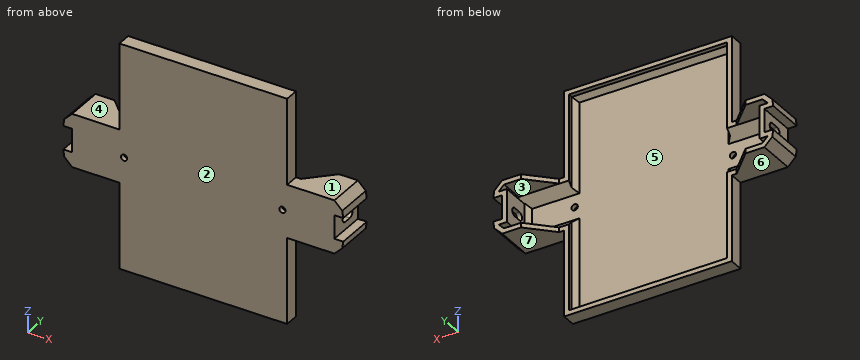
```python
from build123d import *

# Parameters (mm, degrees)
SKETCH4_W                = 90.422573022
SKETCH4_H                = 121.412
BOSS_EXTRUDE2_DEPTH      = 2.54
BOSS_EXTRUDE3_DEPTH      = 2.54
BOSS_EXTRUDE4_DEPTH      = 17.78
SKETCH7_W                = 121.034311438
SKETCH7_H                = 121.412
CUT_EXTRUDE1_DEPTH       = 12.7
CHAMFER1_SIZE            = 12.7
CHAMFER3_SIZE            = 5.08
CHAMFER4_SIZE            = 2.54
M4_START                 = -70.677155719
M4_CLEARANCE_SLOT1_DEPTH = 141.354311438
M3_CLEARANCE_HOLE1_D     = 3.4


# Read off the part's stored shape, not the designer's step: M4 Clearance Slot1
with BuildPart() as part:
    # Sketch4 → Boss-Extrude2 (new body)
    with BuildSketch(Plane(origin=(0, 0, 0), x_dir=(1, 0, 0), z_dir=(0, 1, 0))):
        Rectangle(SKETCH4_W, SKETCH4_H)
    extrude(amount=BOSS_EXTRUDE2_DEPTH)

    # Sketch5 → Boss-Extrude3 (add)
    with BuildSketch(Plane(origin=(0, 0, 0), x_dir=(1, 0, 0), z_dir=(0, 1, 0))):
        Polygon((45.211286511, 14.351), (70.694027546, 14.351), (74.922106204, 10.122921342), (75.452355719, 6.35), (70.677155719, 6.35), (70.677155719, -6.35), (75.452355719, -6.35), (74.922106204, -10.122921342), (70.694027546, -14.351), (45.211286511, -14.351), align=None)
        Polygon((-45.211286511, 14.351), (-45.211286511, -14.351), (-70.694027546, -14.351), (-74.922106204, -10.122921342), (-75.452355719, -6.35), (-70.677155719, -6.35), (-70.677155719, 6.35), (-75.452355719, 6.35), (-74.922106204, 10.122921342), (-70.694027546, 14.351), align=None)
    extrude(amount=BOSS_EXTRUDE3_DEPTH)

    # Sketch6 → Boss-Extrude4 (add)
    with BuildSketch(Plane(origin=(0, 2.54, 0), x_dir=(1, 0, 0), z_dir=(0, 1, 0))):
        Polygon((45.211286511, -60.706), (45.211286511, -14.351), (70.694027546, -14.351), (74.922106204, -10.122921342), (75.452355719, -6.35), (70.677155719, -6.35), (70.677155719, 6.35), (75.452355719, 6.35), (74.922106204, 10.122921342), (70.694027546, 14.351), (45.211286511, 14.351), (45.211286511, 60.706), (-45.211286511, 60.706), (-45.211286511, 14.351), (-70.694027546, 14.351), (-74.922106204, 10.122921342), (-75.452355719, 6.35), (-70.677155719, 6.35), (-70.677155719, -6.35), (-75.452355719, -6.35), (-74.922106204, -10.122921342), (-70.694027546, -14.351), (-45.211286511, -14.351), (-45.211286511, -60.706), align=None)
        Polygon((42.671286511, -58.166), (42.671286511, -11.811), (69.641925098, -11.811), (72.525104647, -8.927820451), (72.530419964, -8.89), (68.137155719, -8.89), (68.137155719, 8.89), (72.530419964, 8.89), (72.525104647, 8.927820451), (69.641925098, 11.811), (42.671286511, 11.811), (42.671286511, 58.166), (-42.671286511, 58.166), (-42.671286511, 11.811), (-69.641925098, 11.811), (-72.525104647, 8.927820451), (-72.530419964, 8.89), (-68.137155719, 8.89), (-68.137155719, -8.89), (-72.530419964, -8.89), (-72.525104647, -8.927820451), (-69.641925098, -11.811), (-42.671286511, -11.811), (-42.671286511, -58.166), align=None, mode=Mode.SUBTRACT)
    extrude(amount=BOSS_EXTRUDE4_DEPTH)

    # Sketch7 → Cut-Extrude1 (cut)
    with BuildSketch(Plane(origin=(0, 20.32, 0), x_dir=(1, 0, 0), z_dir=(0, 1, 0))):
        Rectangle(SKETCH7_W, SKETCH7_H)
    extrude(amount=-CUT_EXTRUDE1_DEPTH, mode=Mode.SUBTRACT)

    # Chamfer1
    chamfer1_edges = [part.edges().sort_by_distance(p)[0] for p in [
        (-60.517155719, 7.62, -13.081),
        (-60.517155719, 7.62, 13.081),
        (60.517155719, 7.62, 13.081),
        (60.517155719, 7.62, -13.081),
    ]]
    chamfer(chamfer1_edges, length=CHAMFER1_SIZE - 0.0001)  # a hair under: the kernel refuses the full size

    # Chamfer3
    chamfer3_edges = [part.edges().sort_by_distance(p)[0] for p in [
        (-56.156605804, 2.54, 11.811),
        (-56.156605804, 2.54, -11.811),
        (56.156605804, 2.54, 11.811),
        (56.156605804, 2.54, -11.811),
    ]]
    chamfer(chamfer3_edges, length=CHAMFER3_SIZE - 0.0001)  # a hair under: the kernel refuses the full size

    # Chamfer4
    chamfer4_edges = [part.edges().sort_by_distance(p)[0] for p in [
        (42.671286511, 2.54, 32.44855),
        (0, 2.54, 58.166),
        (-42.671286511, 2.54, 32.44855),
        (-42.671286511, 2.54, -32.44855),
        (42.671286511, 2.54, -32.44855),
        (0, 2.54, -58.166),
        (-68.137155719, 2.54, 0),
        (68.137155719, 2.54, 0),
    ]]
    chamfer(chamfer4_edges, length=CHAMFER4_SIZE)

    # M4 Clearance Slot1 outline → M4 Clearance Slot1 (cut)
    with BuildSketch(Plane.YZ.offset(M4_START)):
        with BuildLine():
            Line((9.43, -2.25), (13.43, -2.25))
            ThreePointArc((13.43, -2.25), (15.68, 0), (13.43, 2.25))
            Line((13.43, 2.25), (9.43, 2.25))
            ThreePointArc((9.43, 2.25), (7.18, 0), (9.43, -2.25))
        make_face()
    extrude(amount=M4_CLEARANCE_SLOT1_DEPTH, mode=Mode.SUBTRACT)

    # M3 Clearance Hole1 (through all)
    with Locations(Plane(origin=(0, 2.54, 0), x_dir=(1, 0, 0), z_dir=(0, 1, 0))):
        with Locations((42.671286511, 0), (-42.671286511, 0)):
            Hole(M3_CLEARANCE_HOLE1_D / 2)


solid = part.part
```
Model file for the job. Use its own axes, mm. Face numbers are marked on the shaded views. A direction names the side the tool comes from. Give positions to 0.01 mm unless a question says otherwise; leave off trailing zeros. Loops run counter-clockwise (first coordinate to the right, second up) from the corner with the lowest first, then second, coordinate; pieces in that order, holes last. Notation, with made-up numbers: (14.25, -20.5) - (51.25, -20.5) arc R26 cw to (51.25, 8.5) - close; hole circle Ø8 at (4.25, 57.5). An arc over 180 degrees is marked (long way). One line per item, written item: value. Start each with the question number.
1. Slice it at C-C (z = -20). List the corners of the cut face in (x, y).
2. Slice it at A-A (z = 0). List the corners of the cut face in (x, y), plus the area to 3 significant figures.
3. Slice it at B-B (x = -5.5). List the corners of the cut face in (y, z), plus the area to 3 significant figures.
4. Pin check, flat tips, straight feed: pin 1 (12 mm diameter, centred on y = 15.5, z = -1.5, fed in from +X); pin 2 (2.5 mm diameter, centred on x = 74, y = 12.5, fed in from +Z) (3 decimals); pin 3 (1.5 mm diameter, centred on y = 11.5, z = -9.5, fed in from -X). Stop position of each tip, or through.
5. Slice it at D-D (y = 11.25). Give the number of separate pieces and of enclosed holes in the cut face, plus the area to 3 significant figures.
6. Which spindle directions (+Z, -Z, +X, -X, +Y, -Y) get a long thin tool onto all of the face, cutting with end or side? Do the marked faces 4, 5, 6 and 7. Say none if no direction does.
7. Pull direction Z, two halves, no side cores. Call the marked faces 1, 2 and 3: pulls with the +Z half, pulls with the -Z half, needs draft (parallel to the pull), parting line crosses it, or undercut.
8. Probe L1, parallel to X at y = 7, z = 49; L2, parallel to X at y = 12.5, z = -5.5; L3, parallel to Y at x = 1.5, z = -24. List the from-to ranges inside material, lowest first. Write a range as from..to.
Solution:
1. outline: (-45.21, 0) - (45.21, 0) - (45.21, 7.62) - (42.67, 7.62) - (42.67, 5.08) - (40.13, 2.54) - (-40.13, 2.54) - (-42.67, 5.08) - (-42.67, 7.62) - (-45.21, 7.62) - close
2. outline: (-70.68, 0) - (-44.37, 0) - (-44.37, 2.54) - (-65.6, 2.54) - (-68.14, 5.08) - (-68.14, 7.18) - (-70.68, 7.18) - close; (-70.68, 15.68) - (-68.14, 15.68) - (-68.14, 20.32) - (-70.68, 20.32) - close; (-40.97, 0) - (40.97, 0) - (40.97, 2.54) - (-40.97, 2.54) - close; (44.37, 0) - (70.68, 0) - (70.68, 7.18) - (68.14, 7.18) - (68.14, 5.08) - (65.6, 2.54) - (44.37, 2.54) - close; (68.14, 15.68) - (70.68, 15.68) - (70.68, 20.32) - (68.14, 20.32) - close
2. area: 395 mm^2
3. outline: (0, -60.71) - (7.62, -60.71) - (7.62, -58.17) - (5.08, -58.17) - (2.54, -55.63) - (2.54, 55.63) - (5.08, 58.17) - (7.62, 58.17) - (7.62, 60.71) - (0, 60.71) - close
3. area: 341 mm^2
4. pin 1: stops at x = 75.45
4. pin 2: stops at z = 12.295
4. pin 3: stops at x = -75.12
5. separate pieces: 4
5. enclosed holes: 0
5. area: 362 mm^2
6. face 4: +Z, -X, +Y, -Y
6. face 5: +Y
6. face 6: -Z, -X, +Y, -Y
6. face 7: -Z, +X, +Y, -Y
7. face 1: pulls with the +Z half
7. face 2: needs draft
7. face 3: undercut
8. L1: x = -45.21..-42.67, 42.67..45.21
8. L2: x = -70.68..-68.14, 68.14..70.68
8. L3: y = 0..2.54
